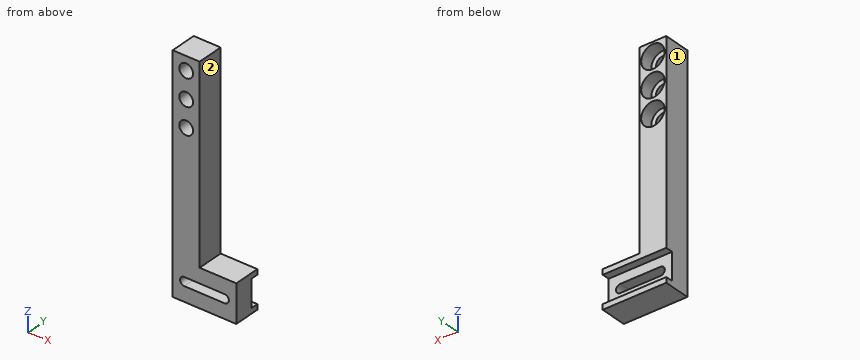
Autodesk Inventor part; units mm, degrees
ref_plane "YZ Plane" through (0, 0, 0) normal (1, 0, 0) x (0, 1, 0)
ref_plane "XZ Plane" through (0, 0, 0) normal (0, 1, 0) x (-1, 0, 0)
ref_plane "XY Plane" through (0, 0, 0) normal (0, 0, 1) x (1, 0, 0)
sketch "Sketch1" plane through (0, 0, 0) normal (0, 1, 0) x (-1, 0, 0)
  line L0 (0, 0) -> (30, 0)
  line L1 (30, 0) -> (30, 108)
  line L2 (30, 108) -> (17.3, 108)
  line L3 (17.3, 108) -> (17.3, 17.8)
  line L4 (17.3, 17.8) -> (0, 17.8)
  line L5 (0, 17.8) -> (0, 0)
  dimension "d0" = 30
  dimension "d1" = 108
  dimension "d2" = 12.7
  dimension "d3" = 90.2
extrude "Extrusion1" add sketch "Sketch1" along normal blind 12.5
sketch "Sketch2" plane through (0, 12.5, 0) normal (0, 1, 0) x (1, 0, 0)
  line L0 (0, -17.8) -> (0, 0)
  line L1 (-30, 0) -> (-30, -108)
  line L2 (-30, 0) -> (-30, -108)
  line L3 (0, -15.3) -> (-30, -15.3)
  line L4 (-30, -15.3) -> (-30, -2.5)
  line L5 (-30, -2.5) -> (0, -2.5)
  line L6 (0, -2.5) -> (0, -15.3)
  dimension "d6" = 12.8
extrude "Extrusion2" cut sketch "Sketch2" against normal blind 3.5
sketch "Sketch3" plane through (0, 9, 0) normal (0, 1, 0) x (1, 0, 0)
  line L0 (-30, -8.9) -> (0, -8.9) construction
  line L1 (0, -17.8) -> (0, 0)
  arc A0 (-5.5, -10.9) -> (-5.5, -6.9) centre (-5.5, -8.9) ccw
  arc A1 (-24.5, -6.9) -> (-24.5, -10.9) centre (-24.5, -8.9) ccw
  line L2 (-24.5, -10.9) -> (-5.5, -10.9)
  line L3 (-5.5, -6.9) -> (-24.5, -6.9)
  dimension "d9" = 4
  dimension "d10" = 4
extrude "Extrusion3" cut sketch "Sketch3" against normal through all
sketch "Sketch4" plane through (0, 12.5, 0) normal (0, 1, 0) x (1, 0, 0)
  line L0 (-30, -108) -> (-17.3, -108)
  line L1 (-23.65, -108) -> (-23.65, -15.5103) construction
  circle A0 centre (-23.65, -101.5) radius 5.5
  circle A1 centre (-23.65, -89) radius 5.5
  circle A2 centre (-23.65, -76.5) radius 5.5
  circle A3 centre (-23.65, -76.5) radius 3.25
  circle A4 centre (-23.65, -89) radius 3.25
  circle A5 centre (-23.65, -101.5) radius 3.25
  point P0 (0, 0)
  dimension "d13" = 11
  dimension "d14" = 11
  dimension "d15" = 11
  dimension "d16" = 12.5
  dimension "d17" = 12.5
  dimension "d18" = 6.5
  dimension "d19" = 6.5
  dimension "d20" = 6.5
  dimension "d25" = 6.5
extrude "Extrusion4" cut sketch "Sketch4" against normal through all contours A3 | A4 | A5
extrude "Extrusion5" cut sketch "Sketch4" against normal blind 6
properties part number "HeadbarHolder" material "Aluminum 6061"
Geometry check sheet. Reference: the model listing, model coordinates, mm. Face numbers are marked on the shaded views. A direction names the side the tool comes from. Round coordinates to 2 decimals unless told otherwise and drop trailing zeros. Order: outer loops, then holes, each group sorted by start corner. A loop starts at its lowest first (then second) coordinate and runs counter-clockwise, first axis right, second up. Notation, with made-up numbers: M 65,-40 L 77,-40 A17 cw 77,-35 Z; hole C 65,-21.75 d10. An arc over 180 degrees is marked long. Write each question's results on one line, items separated by ' | '. Start each with the question number.
1. Go/stop test with flat-tipped pins: P1, Ø5, axis at x = -25.5, z = 56, coming from the -Y side; P2, Ø2, axis at x = -20.5, z = 11.5, coming from the +Y side; P3, Ø6, axis at y = 8, z = 61, coming from the +X side; P4, Ø4.5, axis at x = -13, y = 6.5, coming from the +Z side. Record where each tip stops, or that it passes through.
2. Cross-section at B-B on z = 76.5. Record the boundary of the cut face in (x, y), plus the area to 3 significant figures.
3. Cross-section at C-C on y = 1. Record the boundary of the cut face in (x, z), plus the area to 3 significant figures.
4. Material ranges on L1, parallel to Z at x = -23.65, y = 5; L2, parallel to Z at x = -23.65, y = 9.3; L3, parallel to Z at x = -16.5, y = 8.25, recorded low to high. Write a range as from..to.
5. Cross-section at D-D on z = 8.9. Record the boundary of the cut face in (x, y).
6. Cross-section at A-A on y = 10.5. Record the boundary of the cut face in (x, z).
7. Set-up check for the marked faces 1 and 2: record each of +Z, -Z, +X, -X, +Y, -Y from which the full face is reachable in a straight line by a thin tool's end or side.
Resolved:
1) P1: y = 0 | P2: y = 9 | P3: x = -17.3 | P4: z = 17.8
2) outline: M -30,0 L -26.9,0 L -26.9,6.5 L -29.15,6.5 L -29.15,12.5 L -30,12.5 Z; M -20.4,0 L -17.3,0 L -17.3,12.5 L -18.15,12.5 L -18.15,6.5 L -20.4,6.5 Z | area: 50.5 mm2
3) outline: M -30,0 L 0,0 L 0,17.8 L -17.3,17.8 L -17.3,108 L -30,108 Z; hole C -23.65,76.5 d6.5; hole C -23.65,89 d6.5; hole C -23.65,101.5 d6.5; hole M -24.5,6.9 L -5.5,6.9 A2 ccw -5.5,10.9 L -24.5,10.9 A2 ccw Z | area: 1,490 mm2
4) L1: 0..6.9, 10.9..73.25, 79.75..85.75, 92.25..98.25, 104.75..108 | L2: 0..2.5, 15.3..71, 82..83.5, 94.5..96, 107..108 | L3: 0..6.9, 10.9..17.8
5) outline: M -30,0 L -26.5,0 L -26.5,9 L -30,9 Z; M -3.5,0 L 0,0 L 0,9 L -3.5,9 Z
6) outline: M -30,0 L 0,0 L 0,2.5 L -30,2.5 Z; M -30,15.3 L 0,15.3 L 0,17.8 L -17.3,17.8 L -17.3,108 L -30,108 Z; hole C -23.65,76.5 d11; hole C -23.65,89 d11; hole C -23.65,101.5 d11
7) face 1: +Z, -Z, -X, +Y, -Y | face 2: +Z, +X, +Y, -Y
